Geometry: final body of the model. Coordinates: model frame, mm. Face numbers are marked on the shaded views. A direction names the side the tool comes from. Round coordinates to 2 decimals unless told otherwise and drop trailing zeros. Loops run counter-clockwise (first coordinate to the right, second up) from the corner with the lowest first, then second, coordinate; pieces in that order, holes last. Notation, with made-up numbers: M 73.25,-25.5 L 113.25,-25.5 A19 ccw 113.25,10.5 Z; hole C 83.5,-15.75 d1. An arc over 180 degrees is marked long. Answer as a JSON object with one key per item and string values.
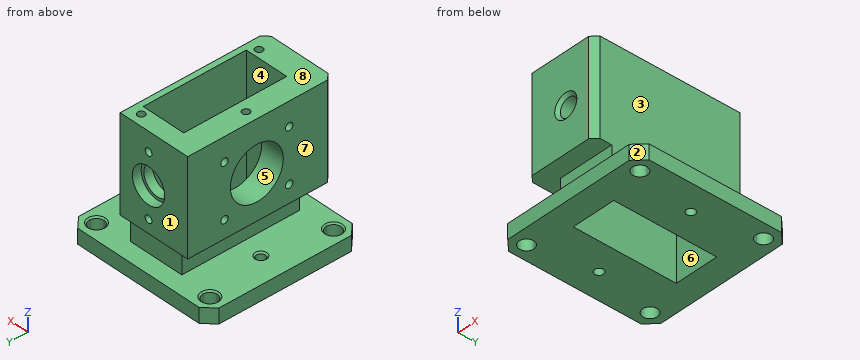
from build123d import *

# Parameters (mm, degrees)
SKETCH_1_W          = 52
SKETCH_1_H          = 52
EXTRUDE_1_DEPTH     = 5
CUT_EXTRUDE_1_DEPTH = 38.107950631
CHAMFER_1_SIZE      = 3.5
CHAMFER_2_SIZE      = 0.5
SKETCH_3_W          = 19
SKETCH_3_H          = 40
EXTRUDE_2_DEPTH     = 42
SKETCH_4_W          = 25
SKETCH_4_H          = 52
EXTRUDE_3_DEPTH     = 32
SKETCH_6_W          = 15
SKETCH_6_H          = 35
CUT_EXTRUDE_2_DEPTH = 60.674114991
CUT_EXTRUDE_3_REACH = 69.877
SKETCH_7_R          = 9
M3X0_51_D           = 2.5
M3X0_51_DEPTH       = 5.5
M3X0_51_TIP         = 0.751075774
CHAMFER_3_SIZE      = 2
M3X0_52_D           = 2.5
M3X0_52_DEPTH       = 5.5
M3X0_52_TIP         = 0.751075774
SKETCH_13_R         = 3.1
CUT_EXTRUDE_4_DEPTH = 7
CUT_EXTRUDE_5_REACH = 72.071
SKETCH_14_R         = 2.05
CHAMFER_4_SIZE      = 1
SKETCH_15_W         = 25
SKETCH_15_H         = 32
CUT_EXTRUDE_6_DEPTH = 2.5
SKETCH_16_R         = 6
CUT_EXTRUDE_7_DEPTH = 3
CUT_EXTRUDE_8_REACH = 73.044
SKETCH_17_R         = 5
M3X0_53_D           = 2.5
M3X0_53_DEPTH       = 4.5
M3X0_53_TIP         = 0.751075774
CUT_EXTRUDE_9_REACH = 61.674
SKETCH_20_R         = 1.5
CHAMFER_5_SIZE      = 0.5


with BuildPart() as part:
    # Эскиз1 → Бобышка-Вытянуть1 (new body)
    with BuildSketch(Plane.XY):
        Rectangle(SKETCH_1_W, SKETCH_1_H)
    extrude(amount=EXTRUDE_1_DEPTH)

    # Эскиз2 → Вырез-Вытянуть1 (cut, through all)
    with BuildSketch(Plane.XY.offset(5)):
        with BuildLine():
            ThreePointArc((-18.5, 21), (-22.767766953, 22.767766953), (-21, 18.5))
            Line((-21, 18.5), (-21, 21))
            Line((-21, 21), (-18.5, 21))
        make_face()
        with BuildLine():
            Line((-21, 21), (-21, 18.5))
            ThreePointArc((-21, 18.5), (-19.232233047, 19.232233047), (-18.5, 21))
            Line((-18.5, 21), (-21, 21))
        make_face()
        with BuildLine():
            ThreePointArc((18.5, 21), (19.232233047, 19.232233047), (21, 18.5))
            Line((21, 18.5), (21, 21))
            Line((21, 21), (18.5, 21))
        make_face()
        with BuildLine():
            Line((21, 21), (21, 18.5))
            ThreePointArc((21, 18.5), (22.767766953, 19.232233047), (23.5, 21))
            ThreePointArc((23.5, 21), (21, 23.5), (18.5, 21))
            Line((18.5, 21), (21, 21))
        make_face()
        with BuildLine():
            Line((-21, -18.5), (-21, -21))
            Line((-21, -21), (-18.5, -21))
            ThreePointArc((-18.5, -21), (-19.232233047, -19.232233047), (-21, -18.5))
        make_face()
        with BuildLine():
            Line((-18.5, -21), (-21, -21))
            Line((-21, -21), (-21, -18.5))
            ThreePointArc((-21, -18.5), (-22.767766953, -22.767766953), (-18.5, -21))
        make_face()
        with BuildLine():
            ThreePointArc((21, -18.5), (19.232233047, -19.232233047), (18.5, -21))
            Line((18.5, -21), (21, -21))
            Line((21, -21), (21, -18.5))
        make_face()
        with BuildLine():
            Line((21, -21), (18.5, -21))
            ThreePointArc((18.5, -21), (21, -23.5), (23.5, -21))
            ThreePointArc((23.5, -21), (22.767766953, -19.232233047), (21, -18.5))
            Line((21, -18.5), (21, -21))
        make_face()
    extrude(amount=-CUT_EXTRUDE_1_DEPTH, mode=Mode.SUBTRACT)

    # Фаска1
    chamfer_1_edges = [part.edges().sort_by_distance(p)[0] for p in [
        (26, -26, 2.5),
        (-26, -26, 2.5),
        (-26, 26, 2.5),
        (26, 26, 2.5),
    ]]
    chamfer(chamfer_1_edges, length=CHAMFER_1_SIZE)

    # Фаска2
    chamfer_2_edges = [part.edges().sort_by_distance(p)[0] for p in [
        (23.5, 21, 5),
        (-21, 23.5, 5),
        (-23.5, -21, 5),
        (18.5, -21, 5),
    ]]
    chamfer(chamfer_2_edges, length=CHAMFER_2_SIZE)

    # Эскиз3 → Бобышка-Вытянуть2 (add)
    with BuildSketch(Plane.XY.offset(5)):
        Rectangle(SKETCH_3_W, SKETCH_3_H)
    extrude(amount=EXTRUDE_2_DEPTH)

    # Эскиз4 → Бобышка-Вытянуть3 (add)
    with BuildSketch(Plane.XY.offset(47)):
        with Locations((-3, 0)):
            Rectangle(SKETCH_4_W, SKETCH_4_H)
    extrude(amount=-EXTRUDE_3_DEPTH)

    # Эскиз6 → Вырез-Вытянуть2 (cut, through all)
    with BuildSketch(Plane.XY.offset(47)):
        Rectangle(SKETCH_6_W, SKETCH_6_H)
    extrude(amount=-CUT_EXTRUDE_2_DEPTH, mode=Mode.SUBTRACT)

    # Эскиз7 → Вырез-Вытянуть3 (cut, up to next)
    with BuildSketch(Plane.ZY.offset(15.5), mode=Mode.PRIVATE) as cut_extrude_3_sk1:
        with Locations((30, 0)):
            Circle(SKETCH_7_R)
    cut_extrude_3_tool1 = extrude(cut_extrude_3_sk1.sketch, amount=-CUT_EXTRUDE_3_REACH, mode=Mode.PRIVATE) & part.part
    add(cut_extrude_3_tool1.solids().sort_by_distance((-15.5, 0, 30))[0], mode=Mode.SUBTRACT)

    # Отверстие обработанное метчиком M3x0.51
    with Locations(Plane(origin=(-15.5, 11, 39), x_dir=(0, 0, -1), z_dir=(-1, 0, 0))):
        with Locations((0, 0), (0, 22), (18, 22), (18, 0)):
            Hole(M3X0_51_D / 2, depth=M3X0_51_DEPTH)
            with Locations((0, 0, -(M3X0_51_DEPTH + M3X0_51_TIP / 2))):  # 118° drill point
                Cone(0, M3X0_51_D / 2, M3X0_51_TIP, mode=Mode.SUBTRACT)

    # Фаска3
    chamfer_3_edges = [part.edges().sort_by_distance(p)[0] for p in [
        (9.5, 26, 31),
        (9.5, -26, 31),
        (-15.5, -26, 31),
        (-15.5, 26, 31),
    ]]
    chamfer(chamfer_3_edges, length=CHAMFER_3_SIZE)

    # Отверстие обработанное метчиком M3x0.52
    with Locations(Plane(origin=(5.5, 20, 47), x_dir=(1, 0, 0), z_dir=(0, 0, 1))):
        with Locations((0, 0), (-17, -20), (0, -40)):
            Hole(M3X0_52_D / 2, depth=M3X0_52_DEPTH)
            with Locations((0, 0, -(M3X0_52_DEPTH + M3X0_52_TIP / 2))):  # 118° drill point
                Cone(0, M3X0_52_D / 2, M3X0_52_TIP, mode=Mode.SUBTRACT)

    # Эскиз13 → Вырез-Вытянуть4 (cut)
    with BuildSketch(Plane(origin=(0, -26, 0), x_dir=(-1, 0, 0), z_dir=(0, -1, 0))):
        with Locations(Location((1, -30, 0), (0, 0, 90))):
            Circle(SKETCH_13_R)
    extrude(amount=-CUT_EXTRUDE_4_DEPTH, mode=Mode.SUBTRACT)

    # Эскиз14 → Вырез-Вытянуть5 (cut, up to next)
    with BuildSketch(Plane.XZ.offset(19), mode=Mode.PRIVATE) as cut_extrude_5_sk1:
        with Locations(Location((-1, 30, 0), (0, 0, 270))):
            Circle(SKETCH_14_R)
    cut_extrude_5_tool1 = extrude(cut_extrude_5_sk1.sketch, amount=-CUT_EXTRUDE_5_REACH, mode=Mode.PRIVATE) & part.part
    add(cut_extrude_5_tool1.solids().sort_by_distance((-1, -19, 30))[0], mode=Mode.SUBTRACT)

    # Фаска4
    chamfer_4_edges = [part.edges().sort_by_distance(p)[0] for p in [
        (-1, -26, 33.1),
    ]]
    chamfer(chamfer_4_edges, length=CHAMFER_4_SIZE)

    # Эскиз15 → Вырез-Вытянуть6 (cut)
    with BuildSketch(Plane(origin=(0, 26, 0), x_dir=(1, 0, 0), z_dir=(0, 1, 0))):
        with Locations((-3, -31)):
            Rectangle(SKETCH_15_W, SKETCH_15_H)
    extrude(amount=-CUT_EXTRUDE_6_DEPTH, mode=Mode.SUBTRACT)

    # Эскиз16 → Вырез-Вытянуть7 (cut)
    with BuildSketch(Plane(origin=(0, 23.5, 0), x_dir=(1, 0, 0), z_dir=(0, 1, 0))):
        with Locations(Location((-1, -30, 0), (0, 0, 270))):
            Circle(SKETCH_16_R)
    extrude(amount=-CUT_EXTRUDE_7_DEPTH, mode=Mode.SUBTRACT)

    # Эскиз17 → Вырез-Вытянуть8 (cut, up to next)
    with BuildSketch(Plane(origin=(0, 20.5, 0), x_dir=(1, 0, 0), z_dir=(0, 1, 0)), mode=Mode.PRIVATE) as cut_extrude_8_sk1:
        with Locations(Location((-1, -30, 0), (0, 0, 270))):
            Circle(SKETCH_17_R)
    cut_extrude_8_tool1 = extrude(cut_extrude_8_sk1.sketch, amount=-CUT_EXTRUDE_8_REACH, mode=Mode.PRIVATE) & part.part
    add(cut_extrude_8_tool1.solids().sort_by_distance((-1, 20.5, 30))[0], mode=Mode.SUBTRACT)

    # Отверстие обработанное метчиком M3x0.53
    with Locations(Plane(origin=(-1, 23.5, 40.5), x_dir=(0, 0, 1), z_dir=(0, 1, 0))):
        with Locations((0, 0), (-21, 0)):
            Hole(M3X0_53_D / 2, depth=M3X0_53_DEPTH)
            with Locations((0, 0, -(M3X0_53_DEPTH + M3X0_53_TIP / 2))):  # 118° drill point
                Cone(0, M3X0_53_D / 2, M3X0_53_TIP, mode=Mode.SUBTRACT)

    # Эскиз20 → Вырез-Вытянуть9 (cut, up to next)
    with BuildSketch(Plane(origin=(0, 0, 0), x_dir=(-1, 0, 0), z_dir=(0, 0, -1)), mode=Mode.PRIVATE) as cut_extrude_9_sk1:
        with Locations((-17, 0)):
            Circle(SKETCH_20_R)
    cut_extrude_9_tool1 = extrude(cut_extrude_9_sk1.sketch, amount=-CUT_EXTRUDE_9_REACH, mode=Mode.PRIVATE) & part.part
    # Эскиз20 → Вырез-Вытянуть9 (cut, up to next)
    with BuildSketch(Plane(origin=(0, 0, 0), x_dir=(-1, 0, 0), z_dir=(0, 0, -1)), mode=Mode.PRIVATE) as cut_extrude_9_sk2:
        with Locations((17, 0)):
            Circle(SKETCH_20_R)
    cut_extrude_9_tool2 = extrude(cut_extrude_9_sk2.sketch, amount=-CUT_EXTRUDE_9_REACH, mode=Mode.PRIVATE) & part.part
    add(cut_extrude_9_tool1.solids().sort_by_distance((17, 0, 0))[0], mode=Mode.SUBTRACT)
    add(cut_extrude_9_tool2.solids().sort_by_distance((-17, 0, 0))[0], mode=Mode.SUBTRACT)

    # Фаска5
    chamfer_5_edges = [part.edges().sort_by_distance(p)[0] for p in [
        (18.5, 0, 5),
        (-15.5, 0, 5),
    ]]
    chamfer(chamfer_5_edges, length=CHAMFER_5_SIZE)


solid = part.part
1) Pin query (flat end, axial travel): P1, Ø12, axis at x = -13.5, z = 26.5, coming from the +Y side; P2, Ø10, axis at y = -14.5, z = 38.5, coming from the -X side; P3, Ø12.5, axis at y = -7.5, z = 18, coming from the +X side; P4, Ø2, axis at x = -17.5, z = 21.5, coming from the +Y side. Return the tip coordinate at first contact, or that it passes through.
Results:
{"P1": "y = 23.5", "P2": "x = -15.5", "P3": "x = 9.5", "P4": "through"}
2) Pull-direction query (X, two-part tool) for the marked faces 6, 7 and 8; classes: +X half, -X half, draft (parallel to the pull), parting line (faces both ways), or undercut.
Results:
{"face 6": "undercut", "face 7": "-X half", "face 8": "draft"}
3) Ray query, line 1 (Z direction, x = -13.6, y = 11); line 2 (X direction, y = -16.5, z = 39.5); line 3 (Y direction, x = 4, z = 33). Return the intervals inside material, ascending.
Results:
{"line 1": "0 to 5, 15 to 19.75, 22.25 to 37.75, 40.25 to 47", "line 2": "-15.5 to -7.5, 7.5 to 9.5", "line 3": "-26 to -17.5, 17.5 to 20.5"}
4) Reachability of the marked faces 1, 2, 3, 4 and 5 from +Z, -Z, +X, -X, +Y, -Y: full face, straight path, thin tool, end or side. Return the list, or none.
Results:
{"face 1": "+Z, +X, -X, +Y", "face 2": "+Z, -Z, +X, -Y", "face 3": "+Z, +X, +Y, -Y", "face 4": "+Z, -Z", "face 5": "-X"}
5) Section query C-C (y = -3). Return the cut outline in (x, z), and give its area (3 significant figures).
Results:
{"outline": "M -26,0 L -7.5,0 L -7.5,21.51 L -15.5,21.51 L -15.5,15 L -9.5,15 L -9.5,5 L -26,5 Z; M -15.5,38.49 L -7.5,38.49 L -7.5,47 L -15.5,47 Z; M 7.5,0 L 26,0 L 26,5 L 9.5,5 L 9.5,47 L 7.5,47 Z", "area": "409 mm2"}
6) Section query A-A (z = 14). Return the cut outline in (x, y), and give its area (3 significant figures).
Results:
{"outline": "M -9.5,-20 L 9.5,-20 L 9.5,20 L -9.5,20 Z; hole M -7.5,-17.5 L 7.5,-17.5 L 7.5,17.5 L -7.5,17.5 Z", "area": "235 mm2"}
7) Section query B-B (x = -17). Return the cut outline in (y, z).
Results:
{"outline": "M -26,0 L -1.5,0 L -1.5,4.5 L -2,5 L -26,5 Z; M 1.5,0 L 26,0 L 26,5 L 2,5 L 1.5,4.5 Z"}
